Part print with two shaded views. Sizes in mm from the minimum x, y, z corner. Round coordinates to 2 decimals unless told otherwise and drop trailing zeros. Order: outer loops, then holes, each group sorted by start corner. A loop starts at its lowest first (then second) coordinate and runs counter-clockwise, first axis right, second up. Notation, with made-up numbers: (36.5, 80) -> (47.5, 80) arc R15 ccw to (47.5, 104) -> close; hole circle Ø6 at (69, -40). An arc over 180 degrees is marked (long way). Put each result on its own line as item: value. Start each with the question number.
Q1. Cut at A-A, the plane y = 25.4. List the corners of the cut face in (x, z) (3 decimals), and give its area (3 significant figures).
Q2. Probe L1, parallel to X at y = 278.5, z = 12.25; L2, parallel to Y at x = 279.4, z = 4.25 (3 decimals); L3, parallel to X at y = 106, z = 11. List the from-to ranges inside material, lowest first.
Q3. Cut at B-B, the plane y = 101.6. List the corners of the cut face in (x, z), and give its area (3 significant figures).
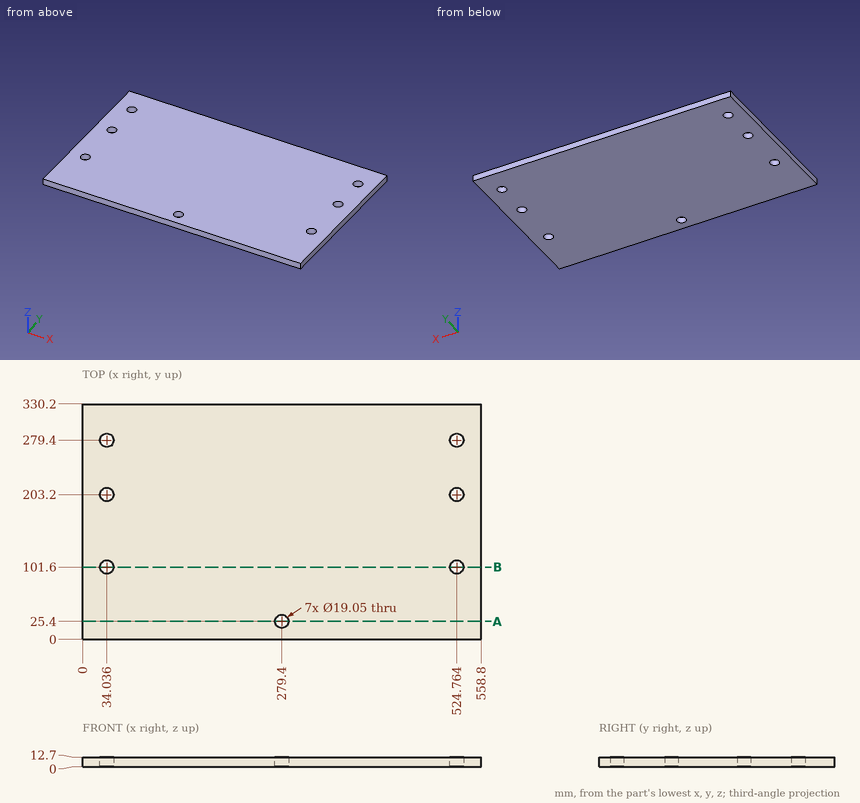
Ans:
1. outline: (0, 0) -> (269.875, 0) -> (269.875, 12.7) -> (0, 12.7) -> close; (288.925, 0) -> (558.8, 0) -> (558.8, 12.7) -> (288.925, 12.7) -> close
1. area: 6,850 mm^2
2. L1: x = 0 to 24.55, 43.52 to 515.28, 534.25 to 558.8
2. L2: y = 0 to 15.875, 34.925 to 330.2
2. L3: x = 0 to 25.59, 42.48 to 516.32, 533.21 to 558.8
3. outline: (0, 0) -> (24.51, 0) -> (24.51, 12.7) -> (0, 12.7) -> close; (43.56, 0) -> (515.24, 0) -> (515.24, 12.7) -> (43.56, 12.7) -> close; (534.29, 0) -> (558.8, 0) -> (558.8, 12.7) -> (534.29, 12.7) -> close
3. area: 6,610 mm^2
